from build123d import *

# Parameters (mm, degrees)
SKETCH1_R           = 3.905
SKETCH1_R_2         = 1.905
BOSS_EXTRUDE1_DEPTH = 6.35
SKETCH2_W           = 0.7
SKETCH2_H           = 0.7
BOSS_EXTRUDE2_DEPTH = 6.35


with BuildPart() as part:
    # Sketch1 → Boss-Extrude1 (new body)
    with BuildSketch(Plane.XY):
        Circle(SKETCH1_R)
        Circle(SKETCH1_R_2, mode=Mode.SUBTRACT)
    extrude(amount=BOSS_EXTRUDE1_DEPTH)

    # Sketch2 → Boss-Extrude2 (add)
    with BuildSketch(Plane(origin=(0, 0, 0), x_dir=(-1, 0, 0), z_dir=(0, 0, -1))):
        with Locations((4.239283353, 0)):
            Rectangle(SKETCH2_W, SKETCH2_H)
        with Locations((-4.239283353, 0)):
            Rectangle(SKETCH2_W, SKETCH2_H)
    extrude(amount=-BOSS_EXTRUDE2_DEPTH)


solid = part.part
For this review, take the finished solid that the model builds, in its own axes (mm). Give positions to 0.01 mm unless a question says otherwise; leave off trailing zeros. Order: outer loops, then holes, each group sorted by start corner. A loop starts at its lowest first (then second) coordinate and runs counter-clockwise, first axis right, second up. Notation, with made-up numbers: M 36.5,55.5 L 51.5,55.5 A36 ccw 51.5,89.5 Z; hole C 10.25,33.5 d6. An arc over 180 degrees is marked long. Answer in a Markdown table with one row per item. Add a question column.
(1) Mouldability with a two-part tool opening along X and no side actions: class faces 1 (the face through (-0.41, -1.86, 3.13)), 2 (the face through (0.081, 3.904, 3.131)), 3 (the face through (-1, -2, 0)) as +X half, -X half, draft (parallel to the pull), parting line (faces both ways), or undercut.
(2) Consider section C-C on y = 0. State the section outline as (x, z) points (3 decimals).
(3) For pin 1 (1.5 mm diameter, centred on x = 1.5, y = -2, fed in from -Z); pin 2 (2 mm diameter, centred on x = 2.5, z = 1.5, fed in from +Y); pin 3 (0.8 mm diameter, centred on x = -4, z = 3, fed in from +Y), all flat-tipped, find the tip position at first contact; note any pin that passes through.
(4) Wall thickness on probe 1 along Y at (x, z) = (0, 4.5) (3 decimals); probe 2 along X at (y, z) = (0.25, 2); probe 3 along Y at (x, z) = (-4, 4.25): over which ranges is each line inside the solid? List them lowest first. Write a range as [from, to].
(5) Consider section B-B on x = 0. State the section outline as (y, z) points (3 decimals).
(6) Consider section A-A on z = 1.5. State the section outline as (x, y) points (3 decimals), and give its area (3 significant figures).
(7) Consider section D-D on x = 3.25. State the section outline as (y, z) points, and give its area (3 significant figures).
Evaluation:
| question | item | result |
|---|---|---|
| 1 | face 1 | undercut |
| 1 | face 2 | parting line |
| 1 | face 3 | draft |
| 2 | outline | M -4.589,0 L -1.905,0 L -1.905,6.35 L -4.589,6.35 Z; M 1.905,0 L 4.589,0 L 4.589,6.35 L 1.905,6.35 Z |
| 3 | pin 1 | stops at z = 0 |
| 3 | pin 2 | stops at y = 3.61 |
| 3 | pin 3 | stops at y = 1.51 |
| 4 | probe 1 | y = [-3.905, -1.905], [1.905, 3.905] |
| 4 | probe 2 | x = [-4.59, -1.89], [1.89, 4.59] |
| 4 | probe 3 | y = [-0.35, 0.35] |
| 5 | outline | M -3.905,0 L -1.905,0 L -1.905,6.35 L -3.905,6.35 Z; M 1.905,0 L 3.905,0 L 3.905,6.35 L 1.905,6.35 Z |
| 6 | outline | M -4.589,-0.35 L -3.889,-0.35 A3.905 ccw 3.889,-0.35 L 4.589,-0.35 L 4.589,0.35 L 3.889,0.35 A3.905 ccw -3.889,0.35 L -4.589,0.35 Z; hole C 0,0 d3.81 |
| 6 | area | 37.5 mm^2 |
| 7 | outline | M -2.16,0 L 2.16,0 L 2.16,6.35 L -2.16,6.35 Z |
| 7 | area | 27.5 mm^2 |
